Work out the finished part from the listing and answer in its coordinate system (mm). A direction names the side the tool comes from. Give positions to 0.01 mm unless a question says otherwise; leave off trailing zeros. Loops run counter-clockwise (first coordinate to the right, second up) from the corner with the lowest first, then second, coordinate; pieces in that order, holes last. Notation, with made-up numbers: M -28.5,37.25 L 11.5,37.25 A12 ccw 11.5,46.25 Z; hole C 75.5,-30.5 d11. An arc over 180 degrees is marked long. Use a Markdown table: item, result.
```python
from build123d import *

# Parameters (mm, degrees)
SKETCH_W     = 40
SKETCH_H     = 40
PAD_DEPTH    = 10
POCKET_DEPTH = 5


with BuildPart() as part:
    # Sketch → Pad (new body)
    with BuildSketch(Plane.XY):
        Rectangle(SKETCH_W, SKETCH_H)
    extrude(amount=PAD_DEPTH)

    # Sketch001 (on Face6 of Pad) → Pocket (cut)
    with BuildSketch(Plane.XY.offset(10)):
        with BuildLine():
            Line((-8, -9), (-8, 11))
            Line((0.5, 11), (-8, 11))
            ThreePointArc((0.5, -1), (6.5, 5), (0.5, 11))
            Line((-1.5, -1), (0.5, -1))
            Line((6.5, -9), (-1.5, -1))
            Line((3, -9), (6.5, -9))
            Line((-5, -1), (3, -9))
            Line((-5, -9), (-5, -1))
            Line((-8, -9), (-5, -9))
        make_face()
        with BuildLine():
            ThreePointArc((0.5, 2), (3.5, 5), (0.5, 8))
            Line((0.5, 8), (-5, 8))
            Line((-5, 8), (-5, 2))
            Line((-5, 2), (0.5, 2))
        make_face(mode=Mode.SUBTRACT)
    extrude(amount=-POCKET_DEPTH, mode=Mode.SUBTRACT)


solid = part.part
```
(1) A cutting plane is placed at A-A (z = 7.25). Write down the section's boundary in (x, y).
Entries:
| item | result |
|---|---|
| outline | M -20,-20 L 20,-20 L 20,20 L -20,20 Z; M -5,2 L 0.5,2 A3 ccw 0.5,8 L -5,8 Z; hole M -8,-9 L -5,-9 L -5,-1 L 3,-9 L 6.5,-9 L -1.5,-1 L 0.5,-1 A6 ccw 0.5,11 L -8,11 Z |
(2) A cutting plane is placed at D-D (y = -8.5). Write down the section's boundary in (x, z).
Entries:
| item | result |
|---|---|
| outline | M -20,0 L 20,0 L 20,10 L 6,10 L 6,5 L 2.5,5 L 2.5,10 L -5,10 L -5,5 L -8,5 L -8,10 L -20,10 Z |
(3) Which of the six approach directions +Z, -Z, +X, -X, +Y, -Y give full straight-line access (tool end or side, diameter ignored) to faces 5 (the flat face through (0, 20, 5)), 6 (the flat face through (-2, 8, 8))?
Entries:
| item | result |
|---|---|
| face 5 | +Z, -Z, +X, -X, +Y |
| face 6 | +Z |
(4) A cutting plane is placed at B-B (y = 5). Write down the section's boundary in (x, z), and give its area (3 significant figures).
Entries:
| item | result |
|---|---|
| outline | M -20,0 L 20,0 L 20,10 L 6.5,10 L 6.5,5 L 3.5,5 L 3.5,10 L -5,10 L -5,5 L -8,5 L -8,10 L -20,10 Z |
| area | 370 mm² |
(5) A cutting plane is placed at C-C (x = -6). Write down the section's boundary in (y, z), and give its area (3 significant figures).
Entries:
| item | result |
|---|---|
| outline | M -20,0 L 20,0 L 20,10 L 11,10 L 11,5 L -9,5 L -9,10 L -20,10 Z |
| area | 300 mm² |
(6) Consider probe 1 along Y at (x, z) = (-4.5, 5.25); probe 2 along X at (y, z) = (-2, 8); probe 3 along Y at (x, z) = (-7.5, 5.25). Determine where each line is inside the solid, lowest interval first. Write a range as [from, to].
Entries:
| item | result |
|---|---|
| probe 1 | y = [-20, -1.5], [2, 8], [11, 20] |
| probe 2 | x = [-20, -8], [-5, -4], [-0.5, 20] |
| probe 3 | y = [-20, -9], [11, 20] |
(7) Given P1, Ø4, axis at x = -3, y = -3.5, coming from the -Z side, flat-ended and moving along its own axis, determine where the tip first touches the part or whether it passes through.
Entries:
| item | result |
|---|---|
| P1 | stops at z = 0 |
(8) The mould has two halves that part along X. Classify faces 1 (the flat face through (20, 0, 5)), 2 (the flat face through (-4.7, -4.2, 10)), 3 (the cylindrical face through (3.5, 4.9, 7.5)), 4 (the flat face through (-2, 2, 8)): released by +X, released by -X, zero draft, split by the parting line, or undercut.
Entries:
| item | result |
|---|---|
| face 1 | released by +X |
| face 2 | zero draft |
| face 3 | undercut |
| face 4 | undercut |
